from build123d import *

# Parameters (mm, degrees)
SKETCH1_R              = 5.207
BOSS_EXTRUDE1_DEPTH    = 3.175
SKETCH2_W              = 65.278
SKETCH2_H              = 25.4
BOSS_EXTRUDE2_DEPTH    = 3.175
FILLET1_R              = 3.175
CONVERT_SOLID1_DEPTH   = 65.278
CONVERT_SOLID1_2_DEPTH = 65.278
CUT_EXTRUDE1_DEPTH     = 104.864417073


# Read off the part's stored shape, not the designer's step: Convert-Solid1
with BuildPart() as part:
    # Sketch1 → Boss-Extrude1 (new body)
    with BuildSketch(Plane.XY):
        with BuildLine():
            Line((0, 0), (65.278, 0))
            Line((65.278, 0), (65.278, 66.802))
            ThreePointArc((65.278, 66.802), (56.515, 75.565), (47.752, 66.802))
            ThreePointArc((47.752, 66.802), (32.639, 51.689), (17.526, 66.802))
            ThreePointArc((17.526, 66.802), (8.763, 75.565), (0, 66.802))
            Line((0, 66.802), (0, 0))
        make_face()
        with Locations((8.763, 66.802)):
            Circle(SKETCH1_R, mode=Mode.SUBTRACT)
        with Locations((56.515, 66.802)):
            Circle(SKETCH1_R, mode=Mode.SUBTRACT)
    extrude(amount=BOSS_EXTRUDE1_DEPTH)

    # Sketch2 → Boss-Extrude2 (add)
    with BuildSketch(Plane(origin=(0, 0, 0), x_dir=(1, 0, 0), z_dir=(0, 1, 0))):
        with Locations((32.639, -15.875)):
            Rectangle(SKETCH2_W, SKETCH2_H)
        with BuildLine():
            Line((16.764, -15.73022), (16.764, -20.81022))
            ThreePointArc((16.764, -20.81022), (12.7, -24.87422), (8.636, -20.81022))
            Line((8.636, -20.81022), (8.636, -15.73022))
            ThreePointArc((8.636, -15.73022), (12.7, -11.66622), (16.764, -15.73022))
        make_face(mode=Mode.SUBTRACT)
        with BuildLine():
            Line((48.514, -15.73022), (48.514, -20.81022))
            ThreePointArc((48.514, -20.81022), (52.578, -24.87422), (56.642, -20.81022))
            Line((56.642, -20.81022), (56.642, -15.73022))
            ThreePointArc((56.642, -15.73022), (52.578, -11.66622), (48.514, -15.73022))
        make_face(mode=Mode.SUBTRACT)
    extrude(amount=BOSS_EXTRUDE2_DEPTH)

    # Fillet1
    fillet1_edges = [part.edges().sort_by_distance(p)[0] for p in [
        (0, 1.5875, 28.575),
        (65.278, 1.5875, 28.575),
    ]]
    fillet(fillet1_edges, radius=FILLET1_R)

    # Convert-Solid1 outline → Convert-Solid1 (cut)
    with BuildSketch(Plane.YZ):
        with BuildLine():
            ThreePointArc((6.35, 0), (1.859871939, 1.859871939), (0, 6.35))
            Line((0, 6.35), (0, 0))
            Line((0, 0), (6.35, 0))
        make_face()
    extrude(amount=CONVERT_SOLID1_DEPTH, mode=Mode.SUBTRACT)

    # Convert-Solid1 2 outline → Convert-Solid1 2 (add)
    with BuildSketch(Plane.YZ):
        with BuildLine():
            ThreePointArc((6.35, 3.175), (4.10493597, 4.10493597), (3.175, 6.35))
            Line((3.175, 6.35), (3.175, 3.175))
            Line((3.175, 3.175), (6.35, 3.175))
        make_face()
    extrude(amount=CONVERT_SOLID1_2_DEPTH)

    # Sketch3 → Cut-Extrude1 (cut, through all)
    with BuildSketch(Plane(origin=(0, 0, 0), x_dir=(-1, 0, 0), z_dir=(0, 0, -1))):
        with BuildLine():
            ThreePointArc((-54.001056047, 19.766894808), (-57.256030763, 19.618085357), (-58.928, 22.41478404))
            Line((-58.928, 22.41478404), (-58.928, 42.164))
            ThreePointArc((-58.928, 42.164), (-57.99806403, 44.40906403), (-55.753, 45.339))
            Line((-55.753, 45.339), (-25.904022132, 45.339))
            ThreePointArc((-25.904022132, 45.339), (-22.863654283, 43.078761359), (-24.152078179, 39.516110768))
            Line((-24.152078179, 39.516110768), (-54.001056047, 19.766894808))
        make_face()
        with BuildLine():
            ThreePointArc((-42.621372005, 12.7), (-45.661739854, 14.960238641), (-44.373315958, 18.522889232))
            Line((-44.373315958, 18.522889232), (-11.276943953, 40.42070433))
            ThreePointArc((-11.276943953, 40.42070433), (-8.021969237, 40.569513781), (-6.35, 37.772815098))
            Line((-6.35, 37.772815098), (-6.35, 15.875))
            ThreePointArc((-6.35, 15.875), (-7.27993597, 13.62993597), (-9.525, 12.7))
            Line((-9.525, 12.7), (-42.621372005, 12.7))
        make_face()
    extrude(amount=-CUT_EXTRUDE1_DEPTH, mode=Mode.SUBTRACT)


solid = part.part
Can you work these out from the model? Positions are in its coordinate system, mm. A direction names the side the tool comes from. Coordinates: 2 decimals unless noted, no trailing zeros. Write each loop counter-clockwise with the first axis right and the second up, starting at its lowest first coordinate (ties: lowest second). Pieces come first, ordered by that corner, then holes. Notation, with made-up numbers: (80.5, 34.25) -> (130.5, 34.25) arc R22 cw to (130.5, 41.25) -> close; hole circle Ø2 at (73, 61.25). An arc over 180 degrees is marked (long way). Write each question's results on one line, items separated by ' | '. Start each with the question number.
Item 1: Thinking about a two-plate mould opening in X: for faces 4 (the flat face through (0, 26, 1)), 5 (the cylindrical face through (57.214, 19.596, 1.565)), 6 (the flat face through (28.057, 29.319, 1.565)), 7 (the flat face through (32, 3.175, 17)), which applies, released by +X, released by -X, zero draft, split by the parting line, or undercut?
Item 2: If we section it at D-D, the plane x = 12.7: Write out the boundary of the cut face in (y, z) (3 decimals), and give its area (3 significant figures).
Item 3: I'm going to push flat-ended pins straight in: P1, Ø2.5, axis at x = 24, z = 2, coming from the +Y side; P2, Ø2.5, axis at x = 41.5, z = 1, coming from the -Y side; P3, Ø13.5, axis at x = 56.515, y = 66.802, coming from the +Z side (3 decimals). Where does each tip first touch, or does it pass through?
Item 4: If we section it at C-C, the plane y = 63: Write out the boundary of the cut face in (x, z) (3 decimals), and give its area (3 significant figures).
Item 5: If we section it at B-B, the plane x = 30: Write out the boundary of the cut face in (y, z) (3 decimals), and give its area (3 significant figures).
Item 6: Please list where these lines run through material, in increasing order: probe 1 along Y at (x, z) = (29, 6.25); probe 2 along Z at (x, y) = (61, 7.5) (3 decimals).
Item 7: If we section it at A-A, the plane y = 27.5: Write out the boundary of the cut face in (x, z) (3 decimals).
Item 8: On a 3-axis mill with a long thin cutter (end or side, diameter ignored), from which of +Z, -Z, +X, -X, +Y, -Y can I reach the whole of each face in a straight line? I mean faces 1 (the flat face through (56.642, 2, 18)), 2 (the cylindrical face through (22.88, 43.13, 1.57)), 3 (the flat face through (32, 34, 3.175)). Say none if no direction works.
Answer block:
1) face 4: released by -X | face 5: undercut | face 6: undercut | face 7: zero draft
2) outline: (0, 6.35) arc R6.35 ccw to (6.35, 0) -> (12.7, 0) -> (12.7, 3.175) -> (6.35, 3.175) arc R3.175 cw to (3.175, 6.35) -> (3.175, 11.666) -> (0, 11.666) -> close; (0, 24.874) -> (3.175, 24.874) -> (3.175, 28.575) -> (0, 28.575) -> close; (39.479, 0) -> (63.394, 0) -> (63.394, 3.175) -> (39.479, 3.175) -> close; (70.21, 0) -> (74.631, 0) -> (74.631, 3.175) -> (70.21, 3.175) -> close | area: 163 mm²
3) P1: y = 55.37 | P2: y = 1.5 | P3: z = 3.175
4) outline: (0, 0) -> (5.205, 0) -> (5.205, 3.175) -> (0, 3.175) -> close; (12.321, 0) -> (18.012, 0) -> (18.012, 3.175) -> (12.321, 3.175) -> close; (47.266, 0) -> (52.957, 0) -> (52.957, 3.175) -> (47.266, 3.175) -> close; (60.073, 0) -> (65.278, 0) -> (65.278, 3.175) -> (60.073, 3.175) -> close | area: 69.2 mm²
5) outline: (0, 6.35) arc R6.35 ccw to (6.35, 0) -> (12.7, 0) -> (12.7, 3.175) -> (6.35, 3.175) arc R3.175 cw to (3.175, 6.35) -> (3.175, 28.575) -> (0, 28.575) -> close; (28.033, 0) -> (35.647, 0) -> (35.647, 3.175) -> (28.033, 3.175) -> close; (45.339, 0) -> (51.921, 0) -> (51.921, 3.175) -> (45.339, 3.175) -> close | area: 160 mm²
6) probe 1: 0 to 3.18 | probe 2: 0 to 3.175
7) outline: (0, 0) -> (6.35, 0) -> (6.35, 3.175) -> (0, 3.175) -> close; (30.805, 0) -> (42.313, 0) -> (42.313, 3.175) -> (30.805, 3.175) -> close; (58.928, 0) -> (65.278, 0) -> (65.278, 3.175) -> (58.928, 3.175) -> close
8) face 1: +Y, -Y | face 2: +Z, -Z | face 3: +Z, +X, -X, +Y
